```python
from build123d import *

# Parameters (mm, degrees)
SKETCH_1_R          = 32.5
EXTRUDE_1_DEPTH     = 0.9
EXTRUDE_START       = -3.9
EXTRUDE_1_2_DEPTH   = 3.9
SKETCH_3_R          = 29
EXTRUDE_2_DEPTH     = 0.9
EXTRUDE_2_2_DEPTH   = 0.9
SKETCH_5_R          = 1.45
SKETCH_5_R_2        = 11.2
CUT_EXTRUDE_1_DEPTH = 3.9


with BuildPart() as part:
    # 草图1 → Extrude 1 (new body)
    with BuildSketch(Plane(origin=(0, 477.404389455, 0), x_dir=(1, 0, 0), z_dir=(0, 1, 0))):
        with Locations(Location((0, 0, 0), (0, 0, 270))):
            Circle(SKETCH_1_R)
    extrude(amount=EXTRUDE_1_DEPTH)

    # 草图2 → Extrude 1 2 (add)
    with BuildSketch(Plane(origin=(0, 478.304389455, 0), x_dir=(1, 0, 0), z_dir=(0, 1, 0)).offset(EXTRUDE_START)):
        with BuildLine():
            ThreePointArc((-32.006251973, -5.643565774), (0, -32.5), (32.006251973, -5.643565774))
            Line((32.006251973, -5.643565774), (32.991059726, -5.817213952))
            ThreePointArc((32.991059726, -5.817213952), (0, -33.5), (-32.991059726, -5.817213952))
            Line((-32.991059726, -5.817213952), (-32.006251973, -5.643565774))
        make_face()
    extrude(amount=EXTRUDE_1_2_DEPTH)



with BuildPart() as body_2:
    # 草图3 → Extrude 2 (new body)
    with BuildSketch(Plane.XZ.offset(-474.404389455)):
        with Locations(Location((0, 0, 0), (0, 0, 270))):
            Circle(SKETCH_3_R)
    extrude(amount=-EXTRUDE_2_DEPTH)


with BuildPart() as part_1:
    add(part.part)

    add(body_2.part)  # Extrude 2 2 merges body 2
    # 草图4 → Extrude 2 2 (add)
    with BuildSketch(Plane.XZ.offset(-474.404389455)):
        with BuildLine():
            ThreePointArc((32.006251973, 5.643565774), (0, 32.5), (-32.006251973, 5.643565774))
            Line((-32.006251973, 5.643565774), (-28.559424837, 5.035797152))
            ThreePointArc((-28.559424837, 5.035797152), (0, 29), (28.559424837, 5.035797152))
            Line((28.559424837, 5.035797152), (32.006251973, 5.643565774))
        make_face()
    extrude(amount=-EXTRUDE_2_2_DEPTH)

    # 草图5 → 切除-拉伸1 (cut)
    with BuildSketch(Plane(origin=(0, 478.304389455, 0), x_dir=(1, 0, 0), z_dir=(0, 1, 0))):
        with Locations(Location((11.545745571, 11.45407173, 0), (0, 0, 270))):
            Circle(SKETCH_5_R)
        with Locations(Location((11.45407173, -11.545745571, 0), (0, 0, 270))):
            Circle(SKETCH_5_R)
        with Locations(Location((-11.545745571, -11.45407173, 0), (0, 0, 270))):
            Circle(SKETCH_5_R)
        with Locations(Location((-11.45407173, 11.545745571, 0), (0, 0, 270))):
            Circle(SKETCH_5_R)
        with Locations(Location((0, 0, 0), (0, 0, 270))):
            Circle(SKETCH_5_R_2)
    extrude(amount=-CUT_EXTRUDE_1_DEPTH, mode=Mode.SUBTRACT)


solid = part_1.part
```
Check sheet for the modelled part. Datum: model origin and axes. Units: mm. A direction names the side the tool comes from. Coordinates: 2 decimals unless noted, no trailing zeros. Write each loop counter-clockwise with the first axis right and the second up, starting at its lowest first coordinate (ties: lowest second). Pieces come first, ordered by that corner, then holes. Notation, with made-up numbers: (81, 58) -> (89, 58) arc R19 ccw to (89, 82) -> close; hole circle Ø4 at (56.25, 40.5). An arc over 180 degrees is marked (long way). Use a Markdown table: item, result.
1. Release check for a two-part mould opening along X. For faces 3 (the cylindrical face through (-12.428, 474.861, 10.303)), 4 (the flat face through (7, 474.404, 10)), 5 (the cylindrical face through (0.79, 477.85, -32.49)), 6 (the cylindrical face through (10.66, 474.86, -12.6)) record: pulls with the +X half, pulls with the -X half, needs draft (parallel to the pull), parting line crosses it, or undercut.
Reported:
| item | result |
|---|---|
| face 3 | undercut |
| face 4 | needs draft |
| face 5 | parting line crosses it |
| face 6 | undercut |
2. Scan lines: line 1 along Y through (x, z) = (2, 21.5); line 2 along X through (y, z) = (477.65, 0); line 3 along Z through (x, y) = (1, 476.8). Record each from-to range of solid material in increasing order.
Reported:
| item | result |
|---|---|
| line 1 | y = 474.4 to 475.3, 477.4 to 478.3 |
| line 2 | x = -32.5 to -11.2, 11.2 to 32.5 |
| line 3 | z = 32.48 to 33.49 |
3. Tool access check on faces 1 (the cylindrical face through (0.655, 476.327, 33.494)), 2 (the flat face through (0, 477.404, 14)). Record the directions out of +Z, -Z, +X, -X, +Y, -Y that give a thin tool (end or side, any length) a straight path to the whole face; none if there is none.
Reported:
| item | result |
|---|---|
| face 1 | +Z, +Y, -Y |
| face 2 | -Z |
4. Go/stop test with flat-tipped pins: pin 1 Ø1.5 at (y, z) = (475, 21.5) entering from +X; pin 2 Ø2 at (y, z) = (475, -20.5) entering from -X. Record where each tip stops, or that it passes through.
Reported:
| item | result |
|---|---|
| pin 1 | stops at x = 26.3 |
| pin 2 | stops at x = -21.47 |
5. Sectioned sample at A-A (x = 0). Enter the section's corners in (y, z).
Reported:
| item | result |
|---|---|
| outline | (474.4, -29) -> (475.3, -29) -> (475.3, -11.2) -> (474.4, -11.2) -> close; (474.4, 11.2) -> (475.3, 11.2) -> (475.3, 32.5) -> (477.4, 32.5) -> (477.4, 11.2) -> (478.3, 11.2) -> (478.3, 33.5) -> (474.4, 33.5) -> close; (477.4, -32.5) -> (478.3, -32.5) -> (478.3, -11.2) -> (477.4, -11.2) -> close |
6. Sectioned sample at B-B (z = 0). Enter the section's corners in (x, y), plus the area to 3 significant figures.
Reported:
| item | result |
|---|---|
| outline | (-32.5, 477.4) -> (-11.2, 477.4) -> (-11.2, 478.3) -> (-32.5, 478.3) -> close; (-29, 474.4) -> (-11.2, 474.4) -> (-11.2, 475.3) -> (-29, 475.3) -> close; (11.2, 474.4) -> (29, 474.4) -> (29, 475.3) -> (11.2, 475.3) -> close; (11.2, 477.4) -> (32.5, 477.4) -> (32.5, 478.3) -> (11.2, 478.3) -> close |
| area | 70.4 mm2 |
7. Sectioned sample at C-C (z = -21.5). Enter the section's corners in (x, y).
Reported:
| item | result |
|---|---|
| outline | (-24.37, 477.4) -> (24.37, 477.4) -> (24.37, 478.3) -> (-24.37, 478.3) -> close; (-19.46, 474.4) -> (19.46, 474.4) -> (19.46, 475.3) -> (-19.46, 475.3) -> close |
8. Sectioned sample at D-D (x = -21.5). Enter the section's corners in (y, z).
Reported:
| item | result |
|---|---|
| outline | (474.4, -19.46) -> (475.3, -19.46) -> (475.3, 24.37) -> (477.4, 24.37) -> (477.4, -24.37) -> (478.3, -24.37) -> (478.3, 25.69) -> (474.4, 25.69) -> close |
